```python
from build123d import *

# Parameters (mm, degrees)
F1_DEPTH = 289.052
F2_T     = -3.556
F4_DEPTH = 3.556


with BuildPart() as f1:
    # F0 (on Right) → F1 (new body, symmetric)
    with BuildSketch(Plane.YZ):
        Polygon((-101.6, 0), (0, 0), (0, 277.876), (-101.6, 176.276), align=None)
    extrude(amount=F1_DEPTH, both=True)

    # F2
    f2_openings = [f1.faces().sort_by_distance(p)[0] for p in [
        (0, 0, 138.938),
        (0, -50.8, 0),
    ]]
    offset(amount=F2_T, openings=f2_openings)

    # F3 (on face) → F4 (join)
    with BuildSketch(Plane(origin=(0, 0, 0), x_dir=(-1, 0, 0), z_dir=(0, 1, 0))):
        Polygon((289.052, 277.876), (-289.052, 277.876), (-289.052, 0), (-273.175836, 0), (-273.175836, 247.904), (273.05, 247.904), (273.05, 0), (289.052, 0), align=None)
    extrude(amount=F4_DEPTH)


solid = f1.part
```
The model under review builds one solid part; all positions refer to its coordinate system, in mm. A direction names the side the tool comes from. Round coordinates to 2 decimals unless told otherwise and drop trailing zeros. Loops run counter-clockwise (first coordinate to the right, second up) from the corner with the lowest first, then second, coordinate; pieces in that order, holes last. Notation, with made-up numbers: M 76.25,29.5 L 127.25,29.5 A20 cw 127.25,54.5 Z; hole C -1.5,23 d3. An arc over 180 degrees is marked long. Write item = value, one per line.
Item 1: The part is to be moulded in two halves that separate along Y. For faces 3 (the flat face through (4, -101.6, 89)), 4 (the flat face through (-289.052, -50, 106)), 5 (the flat face through (-285.496, -50, 108)), say which applies: released by +Y, released by -Y, zero draft, split by the parting line, or undercut.
Return value:
face_3 = released by -Y
face_4 = zero draft
face_5 = undercut
Item 2: Take a section at B-B on z = 165. Write out the cut boundary in (x, y), then the cut area to 3 significant figures.
Return value:
outline = M -289.05,-101.6 L 289.05,-101.6 L 289.05,3.56 L 273.18,3.56 L 273.18,0 L 285.5,0 L 285.5,-98.04 L -285.5,-98.04 L -285.5,0 L -273.05,0 L -273.05,3.56 L -289.05,3.56 Z
area = 2,870 mm2
Item 3: Insertion check: P1, Ø2, axis at x = 73.5, z = 185.5, coming from the +Y side; P2, Ø5, axis at x = -23.5, y = -46.5, coming from the -Z side; P3, Ø8, axis at x = 228.5, y = -42.5, coming from the +Z side. Each pin has a flat end and moves straight along its axis. Give the tip position at first contact, or say it passes through.
Return value:
P1 = -86.35
P2 = 223.85
P3 = 239.38
Item 4: Take a section at C-C on y = -38.5. Write out the cut boundary in (x, z).
Return value:
outline = M -289.05,0 L -285.5,0 L -285.5,234.35 L 285.5,234.35 L 285.5,0 L 289.05,0 L 289.05,239.38 L -289.05,239.38 Z
Item 5: Machinability: for faces 1 (the flat face through (4.047, -50.089, 227.787)), 2 (the flat face through (285.496, -50, 108)), which of the approach directions +Z, -Z, +X, -X, +Y, -Y give a long, thin tool a straight path to every point of the face, cutting with its end or side? Answer none if there is none.
Return value:
face_1 = +Z, +X, -X, -Y
face_2 = -Z
Item 6: Take a section at A-A on x = -226.5. Write out the cut boundary in (y, z).
Return value:
outline = M -101.6,0 L -98.04,0 L -98.04,174.8 L 0,272.85 L 0,247.9 L 3.56,247.9 L 3.56,277.88 L 0,277.88 L -101.6,176.28 Z
Item 7: Take a section at D-D on y = -88. Write out the cut boundary in (x, z), then the cut area to 3 significant figures.
Return value:
outline = M -289.05,0 L -285.5,0 L -285.5,184.85 L 285.5,184.85 L 285.5,0 L 289.05,0 L 289.05,189.88 L -289.05,189.88 Z
area = 4,220 mm2
Item 8: For line 1 (X direction, y = -19, z = 85); line 2 (Y direction, x = 216, z = 32); line 3 (Y direction, x = -89, z = 249), list the stretches that pass through material, from the lowest coordinate up. Write a range as [from, to].
Return value:
line_1 = [-289.05, -285.5], [285.5, 289.05]
line_2 = [-101.6, -98.04]
line_3 = [-28.88, -23.85], [0, 3.56]
